Design review of the part shown in the three views and the two pictorial views. Dimensions are in mm from the part's minimum x, y and z. Round coordinates to 2 decimals unless told otherwise and drop trailing zeros. Write each loop counter-clockwise with the first axis right and the second up, starting at its lowest first coordinate (ties: lowest second). Pieces come first, ordered by that corner, then holes. Notation, with made-up numbers: (7, -39.5) - (36, -39.5) arc R10 ccw to (36, -30.5) - close; hole circle Ø4 at (47.5, 79). An arc over 180 degrees is marked (long way). Use one line per item in the form item = value.
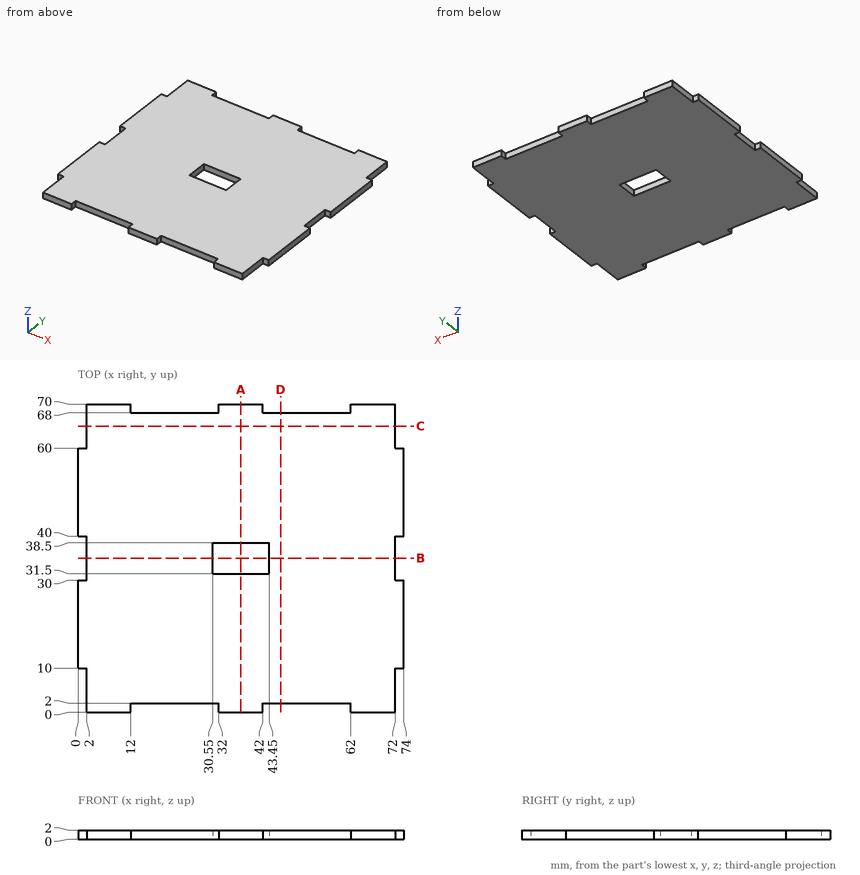
Q1. To check wall thickness, follow line 1 along X through (y, z) = (32, 1.35); line 2 along Y through (x, z) = (33, 0.85); line 3 along X through (y, z) = (5.5, 1). State the ranges of each line that lie inside material, in increasing order. Write a range as from..to.
Calculated:
line_1 = 2..30.55, 43.45..72
line_2 = 0..31.5, 38.5..70
line_3 = 2..72
Q2. We need section D-D on x = 46. Write out the cut boundary in (y, z).
Calculated:
outline = (2, 0) - (68, 0) - (68, 2) - (2, 2) - close
Q3. We need section A-A on x = 37. Write out the cut boundary in (y, z).
Calculated:
outline = (0, 0) - (31.5, 0) - (31.5, 2) - (0, 2) - close; (38.5, 0) - (70, 0) - (70, 2) - (38.5, 2) - close
Q4. For P1, Ø0.6, axis at y = 1, z = 0.5, coming from the +X side; P2, Ø0.6, axis at y = 34, z = 0.5, coming from the -X side, all flat-tipped, find the tip position at first contact; note any pin that passes through.
Calculated:
P1 = 72
P2 = 2
Q5. We need section B-B on y = 35. Write out the cut boundary in (x, z), then the cut area to 3 significant figures.
Calculated:
outline = (2, 0) - (30.55, 0) - (30.55, 2) - (2, 2) - close; (43.45, 0) - (72, 0) - (72, 2) - (43.45, 2) - close
area = 114 mm2
Q6. We need section C-C on y = 65. Write out the cut boundary in (x, z).
Calculated:
outline = (2, 0) - (72, 0) - (72, 2) - (2, 2) - close
